Geometry: final body of the model. Coordinates: model frame, mm. Face numbers are marked on the shaded views. Give positions to 0.01 mm unless a question says otherwise; leave off trailing zeros. Write each loop counter-clockwise with the first axis right and the second up, starting at its lowest first coordinate (ties: lowest second). Pieces come first, ordered by that corner, then holes.
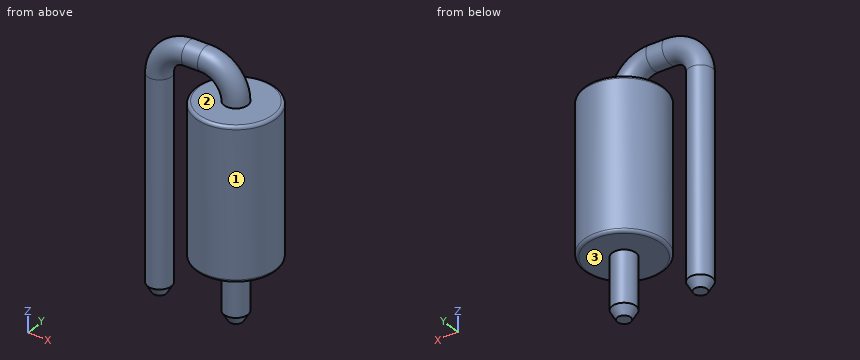
from build123d import *
from OCP.BRepFilletAPI import BRepFilletAPI_MakeChamfer

# Parameters (mm, degrees)
SKETCH1_R      = 0.3937
CHAMFER1_SIZE  = 0.3
CHAMFER1_SIZE2 = 0.173205081
SKETCH4_R      = 1.3335
EXTRUDE2_DEPTH = 5
FILLET2_R      = 0.1


with BuildPart() as part:
    # Sweep1: sweep along a path in Sketch3
    with BuildLine(Plane(origin=(0, 0, 0), x_dir=(1, 0, 0), z_dir=(0, 1, 0))) as sweep1_path:
        Line((1.27, 0), (1.27, -7))
        ThreePointArc((1.27, -7), (0.977106781, -7.707106781), (0.27, -8))
        Line((0.27, -8), (-0.27, -8))
        ThreePointArc((-0.27, -8), (-0.977106781, -7.707106781), (-1.27, -7))
        Line((-1.27, -7), (-1.27, 0))
    # Sketch1 → Sweep1 (sweep)
    with BuildSketch(Plane.XY):
        with Locations((1.27, 0)):
            Circle(SKETCH1_R)
    sweep(path=sweep1_path.line)

    # Chamfer1: one chamfer whose edges measure the first distance from different faces: ONE call of the kernel's chamfer builder (chamfer() names one face for all edges)
    chamfer1_edges_1 = [part.edges().sort_by_distance(p)[0] for p in [
        (0.8763, 0, 0),
    ]]
    chamfer1_side_1 = [part.faces().sort_by_distance(p)[0] for p in [
        (0.8763, 0, 3.5),
    ]]
    chamfer1_edges_2 = [part.edges().sort_by_distance(p)[0] for p in [
        (-0.8763, 0, 0),
    ]]
    chamfer1_side_2 = [part.faces().sort_by_distance(p)[0] for p in [
        (-0.8763, 0, 3.5),
    ]]
    chamfer1 = BRepFilletAPI_MakeChamfer(part.part.solid().wrapped)
    for e in chamfer1_edges_1:
        chamfer1.Add(CHAMFER1_SIZE, CHAMFER1_SIZE2, e.wrapped, chamfer1_side_1[0].wrapped)  # the first distance lies on this face
    for e in chamfer1_edges_2:
        chamfer1.Add(CHAMFER1_SIZE, CHAMFER1_SIZE2, e.wrapped, chamfer1_side_2[0].wrapped)  # the first distance lies on this face
    add(Compound.cast(chamfer1.Shape()), mode=Mode.REPLACE)

    # Sketch4 → Extrude2 (add)
    with BuildSketch(Plane.XY.offset(2)):
        with Locations((1.27, 0)):
            Circle(SKETCH4_R)
    extrude(amount=EXTRUDE2_DEPTH)

    # Fillet2
    fillet2_edges = [part.edges().sort_by_distance(p)[0] for p in [
        (-0.0635, 0, 7),
        (-0.0635, 0, 2),
    ]]
    fillet(fillet2_edges, radius=FILLET2_R)


solid = part.part
Q1. Pin query (flat end, axial travel): P1, Ø2, axis at x = -0.5, z = 4.5, coming from the +Y side. Return the tip coordinate at first contact, or that it passes through.
Filled sheet:
P1: stops at y = 1.09
Q2. Section B-B on y = 0. Output: boundary loops of the cut face in (x, z), plus the area to 3 significant figures.
Filled sheet:
outline: (-1.66, 0.3) - (-1.49, 0) - (-1.05, 0) - (-0.88, 0.3) - (-0.88, 7) arc R0.61 cw to (-0.27, 7.61) - (0.27, 7.61) arc R0.61 cw to (0.88, 7) - (0.04, 7) arc R0.1 ccw to (-0.06, 6.9) - (-0.06, 2.1) arc R0.1 ccw to (0.04, 2) - (0.88, 2) - (0.88, 0.3) - (1.05, 0) - (1.49, 0) - (1.66, 0.3) - (1.66, 2) - (2.5, 2) arc R0.1 ccw to (2.6, 2.1) - (2.6, 6.9) arc R0.1 ccw to (2.5, 7) - (1.66, 7) arc R1.39 ccw to (0.27, 8.39) - (-0.27, 8.39) arc R1.39 ccw to (-1.66, 7) - close
area: 23.2 mm2
Q3. Ray query, line 1 along Z through (x, y) = (2.2, -0.05); line 2 along Y through (x, z) = (-1.3, 2); line 3 along Y through (x, z) = (1.2, 3). Return the intervals inside material, ascending.
Filled sheet:
line 1: z = 2 to 7
line 2: y = -0.39 to 0.39
line 3: y = -1.33 to 1.33
Q4. Section A-A on z = 6.5. Output: boundary loops of the cut face in (x, y), plus the area to 3 significant figures.
Filled sheet:
outline: circle Ø0.79 at (-1.27, 0); circle Ø2.67 at (1.27, 0)
area: 6.07 mm2
Q5. Section C-C on z = 1.5. Output: boundary loops of the cut face in (x, y), plus the area to 3 significant figures.
Filled sheet:
outline: circle Ø0.79 at (-1.27, 0); circle Ø0.79 at (1.27, 0)
area: 0.974 mm2
Q6. Pull-direction query (Z, two-part tool) for the marked faces 1, 2 and 3; classes: released by +Z, released by -Z, zero draft, split by the parting line, or undercut.
Filled sheet:
face 1: zero draft
face 2: undercut
face 3: released by -Z
